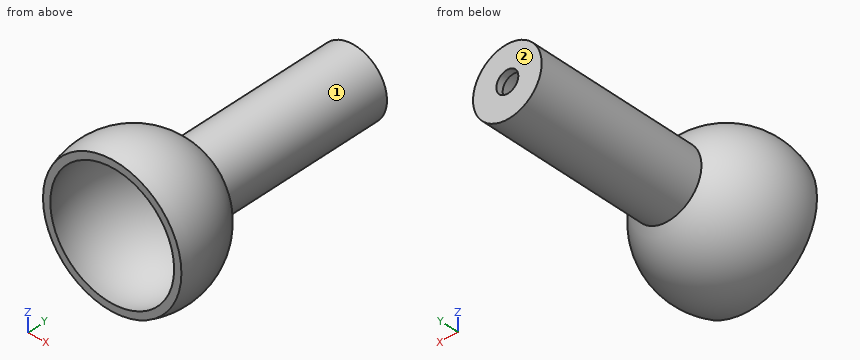
```python
from build123d import *

# Parameters (mm, degrees)
ESBO_O1_R                = 5
RESSALTO_EXTRUS_O1_DEPTH = 30
RESSALTO_EXTRUS_O4_START = -74
ESBO_O4_R                = 5
RESSALTO_EXTRUS_O4_DEPTH = 74
ESBO_O3_R                = 71.162261847
CORTE_EXTRUS_O2_DEPTH    = 36
CORTE_EXTRUS_O3_REACH    = 42.863
ESBO_O6_R                = 1.6


# Read off the part's stored shape, not the designer's step: Domo1, Casca3
with BuildPart() as part:
    # Esboço1 → Ressalto-extrusão1 (new body)
    with BuildSketch(Plane(origin=(0, 0, 0), x_dir=(1, 0, 0), z_dir=(0, 1, 0))):
        with Locations(Location((0, 0, 0), (0, 0, 270))):
            Circle(ESBO_O1_R)
    extrude(amount=-RESSALTO_EXTRUS_O1_DEPTH)

    # Domo1 outline → Domo1 (revolve)
    with BuildSketch(Plane.XY):
        with BuildLine():
            Line((0, 0), (4.999999996, -3e-09))
            ThreePointArc((4.999999996, -3e-09), (10.307764064, 11.951941013), (0, 20))
            Line((0, 20), (0, 0))
        make_face()
    revolve(axis=Axis((0, 0, 0), (0, 1, 0)))

    # Esboço4 → Ressalto-extrusão4 (add)
    with BuildSketch(Plane.XZ.offset(30).offset(RESSALTO_EXTRUS_O4_START)):
        with Locations(Location((0, 0, 0), (0, 0, 90))):
            Circle(ESBO_O4_R)
    extrude(amount=RESSALTO_EXTRUS_O4_DEPTH)

    # Esboço3 → Corte-extrusão2 (cut)
    with BuildSketch(Plane.XZ.offset(30)):
        Circle(ESBO_O3_R)
    extrude(amount=-CORTE_EXTRUS_O2_DEPTH, mode=Mode.SUBTRACT)

    # Casca3 outline → Casca3 (revolve, cut)
    with BuildSketch(Plane.XY):
        with BuildLine():
            Line((3.999999997, 18.129463148), (4, 43))
            Line((4, 43), (0, 43))
            Line((0, 43), (0, 5.999999991))
            Line((0, 5.999999991), (9.013878185, 5.999999991))
            ThreePointArc((9.013878185, 5.999999991), (8.895011268, 13.051873609), (3.999999997, 18.129463148))
        make_face()
    revolve(axis=Axis((0, 0, 0), (0, 1, 0)), mode=Mode.SUBTRACT)

    # Esboço6 → Corte-extrusão3 (cut, up to next)
    with BuildSketch(Plane(origin=(0, 44, 0), x_dir=(1, 0, 0), z_dir=(0, 1, 0)), mode=Mode.PRIVATE) as corte_extrus_o3_sk1:
        with Locations(Location((0, 0, 0), (0, 0, 270))):
            Circle(ESBO_O6_R)
    corte_extrus_o3_tool1 = extrude(corte_extrus_o3_sk1.sketch, amount=-CORTE_EXTRUS_O3_REACH, mode=Mode.PRIVATE) & part.part
    add(corte_extrus_o3_tool1.solids().sort_by_distance((0, 44, 0))[0], mode=Mode.SUBTRACT)


solid = part.part
```
CAD build for the part. Positions are in the model's coordinates, mm. Face numbers are marked on the shaded views. A direction names the side the tool comes from. Give positions to 0.01 mm unless a question says otherwise; leave off trailing zeros. Write each loop counter-clockwise with the first axis right and the second up, starting at its lowest first coordinate (ties: lowest second). Pieces come first, ordered by that corner, then holes. Notation, with made-up numbers: (-23, 83.25) -> (2, 83.25) arc R9 ccw to (2, 91.25) -> close; hole circle Ø3 at (25, -4.5). An arc over 180 degrees is marked (long way). Write each question's results on one line, items separated by ' | '.
1. Cut at B-B, the plane x = 0. Write the cut outline in (y, z) (3 decimals), then the cut area to 3 significant figures.
Geometry check:
outline: (6, -10.075) arc R10.625 ccw to (18.75, -5) -> (44, -5) -> (44, -1.6) -> (43, -1.6) -> (43, -4) -> (18.129, -4) arc R9.625 cw to (6, -9.014) -> close; (6, 9.014) arc R9.625 cw to (18.129, 4) -> (43, 4) -> (43, 1.6) -> (44, 1.6) -> (44, 5) -> (18.75, 5) arc R10.625 ccw to (6, 10.075) -> close | area: 85.3 mm²
2. Wall check: probe 1 along X at (y, z) = (35, 0); probe 2 along X at (y, z) = (43.4, 0); probe 3 along Z at (x, y) = (1.75, 42.5). Give the ranges that are in metal, low to high. Write a range as [from, to].
Geometry check:
probe 1: [-5, -4], [4, 5] | probe 2: [-5, -1.6], [1.6, 5] | probe 3: [-4.68, -3.6], [3.6, 4.68]
3. Cut at C-C, the plane y = 41.5. Write the cut outline in (x, z).
Geometry check:
outline: circle Ø10 at (0, 0); hole circle Ø8 at (0, 0)
4. Which spindle directions (+Z, -Z, +X, -X, +Y, -Y) get a long thin tool onto all of the face, cutting with end or side? Do the marked faces 1 and 2. Say none if no direction does.
Geometry check:
face 1: +Y | face 2: +Z, -Z, +X, -X, +Y
5. Drop flat-ended pins along their axis: P1, Ø8, axis at y = 38, z = -4.5, coming from the -X side; P2, Ø10, axis at x = -3.5, y = 31.5, coming from the -Z side; P3, Ø9, axis at x = 0, z = -1, coming from the -Y side. Give the stop position or say it passes through.
Geometry check:
P1: x = -4.97 | P2: z = -5 | P3: y = 17.27
6. Cut at A-A, the plane z = 0. Write the cut outline in (x, y) (3 decimals), then the cut area to 3 significant figures.
Geometry check:
outline: (-10.075, 6) -> (-9.014, 6) arc R9.625 cw to (-4, 18.129) -> (-4, 43) -> (-1.6, 43) -> (-1.6, 44) -> (-5, 44) -> (-5, 18.75) arc R10.625 ccw to start; (1.6, 43) -> (4, 43) -> (4, 18.129) arc R9.625 cw to (9.014, 6) -> (10.075, 6) arc R10.625 ccw to (5, 18.75) -> (5, 44) -> (1.6, 44) -> close | area: 85.3 mm²
7. Cut at D-D, the plane x = -2.25. Write the cut outline in (y, z) (3 decimals).
Geometry check:
outline: (6, -9.82) arc R10.384 ccw to (18.75, -4.465) -> (44, -4.465) -> (44, 4.465) -> (18.75, 4.465) arc R10.384 ccw to (6, 9.82) -> (6, 8.729) arc R9.358 cw to (18.129, 3.307) -> (43, 3.307) -> (43, -3.307) -> (18.129, -3.307) arc R9.358 cw to (6, -8.729) -> close
